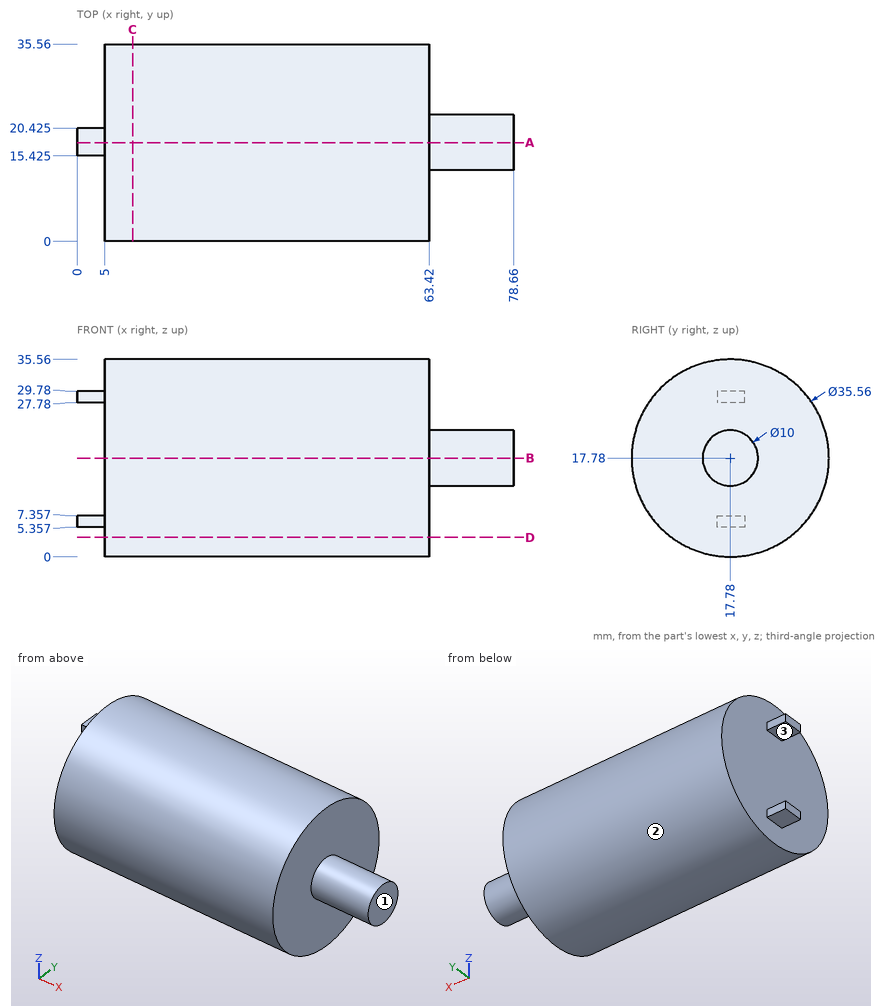
Can you work these out from the drawing? Everything is in mm from the part's minimum corner. Round coordinates to 2 decimals unless told otherwise and drop trailing zeros. Write each loop counter-clockwise with the first axis right and the second up, starting at its lowest first coordinate (ties: lowest second). Pieces come first, ordered by that corner, then holes.
1. Suppose I cut it at C-C (x = 10). List the corners of the cut face in (y, z) for me, and give its area (3 significant figures).
2. If we mould it in two halves opening along Z, with no side actions, what happens to the marked faces 1, 2 and 3? For each: released by +Z, released by -Z, zero draft, split by the parting line, or undercut.
3. Suppose I cut it at B-B (z = 17.78). List the corners of the cut face in (x, y) for me, and give its area (3 significant figures).
4. I need wall thicknesses on L1, parallel to X at y = 7.5, z = 6; L2, parallel to Y at x = 45, z = 17.5. Which ranges of each line are inside material? Lowest first, please.
5. Suppose I cut it at D-D (z = 3.5). List the corners of the cut face in (x, y) for me, and give its area (3 significant figures).
6. Will these pins go through, and if not, where does the flat tip stop? pin 1 Ø1.5 at (x, y) = (2, 19) entering from +Z; pin 2 Ø10 at (y, z) = (11, 25.5) entering from +X; pin 3 Ø4 at (x, y) = (62, 16) entering from +Z; pin 4 Ø3 at (x, z) = (50, 25.5) entering from -Y.
7. Suppose I cut it at A-A (y = 17.78). List the corners of the cut face in (x, z) for me.
Answer sheet:
1. outline: circle Ø35.56 at (17.78, 17.78)
1. area: 993 mm2
2. face 1: zero draft
2. face 2: split by the parting line
2. face 3: undercut
3. outline: (5, 0) - (63.42, 0) - (63.42, 12.78) - (78.66, 12.78) - (78.66, 22.78) - (63.42, 22.78) - (63.42, 35.56) - (5, 35.56) - close
3. area: 2,230 mm2
4. L1: x = 5 to 63.42
4. L2: y = 0 to 35.56
5. outline: (5, 7.19) - (63.42, 7.19) - (63.42, 28.37) - (5, 28.37) - close
5. area: 1,240 mm2
6. pin 1: stops at z = 29.78
6. pin 2: stops at x = 63.42
6. pin 3: stops at z = 35.56
6. pin 4: stops at y = 1.12
7. outline: (0, 5.36) - (5, 5.36) - (5, 0) - (63.42, 0) - (63.42, 12.78) - (78.66, 12.78) - (78.66, 22.78) - (63.42, 22.78) - (63.42, 35.56) - (5, 35.56) - (5, 29.78) - (0, 29.78) - (0, 27.78) - (5, 27.78) - (5, 7.36) - (0, 7.36) - close
